Verification items for the finished model (mm, model axes). A direction names the side the tool comes from. Round coordinates to 2 decimals unless told otherwise and drop trailing zeros. Order: outer loops, then holes, each group sorted by start corner. A loop starts at its lowest first (then second) coordinate and runs counter-clockwise, first axis right, second up. Notation, with made-up numbers: (-21, 72.5) -> (34, 72.5) arc R24 ccw to (34, 85.5) -> close; hole circle Ø8 at (83.25, -13.5). An arc over 180 degrees is marked (long way). Return JSON: item names as keys, results as strings. Group by question number.
1) Section check A-A on x = 0. Enter the section's corners in (y, z).
2) Depth check by flat-ended pin: pin 1 (6 mm diameter, centred on y = -4.5, z = 8.5, fed in from -X); pin 2 (2.5 mm diameter, centred on x = -9, y = -0.5, fed in from +Z); pin 3 (0.8 mm diameter, centred on y = -9.5, z = 9.5, fed in from -X). Enter the tip coordinate at first touch or a pass-through.
3) Draft check along Y on faces 4 (the cylindrical face through (1.9, 11.59, 7.57)), 5 (the cylindrical face through (-3.47, -15.62, 4.45)), 6 (the flat face through (-11, -1, 7)). Enter one of: pulls with the +Y half, pulls with the -Y half, needs draft (parallel to the pull), parting line crosses it, or undercut.
4) Scan lines: L1, parallel to Y at x = 0, z = 3; L2, parallel to X at y = -1, z = 5.75; L3, parallel to X at y = -1, z = 8.75. Record each from-to range of solid material in increasing order.
5) Tool access check on faces 1 (the cylindrical face through (-12.5, 0.1, 8.5)), 2 (the cylindrical face through (-11, 0, 4)), 3 (the flat face through (-2.5, -11.4, 9.5)). Record the directions out of +Z, -Z, +X, -X, +Y, -Y that give a thin tool (end or side, any length) a straight path to the whole face; none if there is none.
6) Section check B-B on z = 7.5. Enter the section's corners in (x, y).
```python
from build123d import *

# Parameters (mm, degrees)
SKETCH_R        = 16
SKETCH_R_2      = 7.5
PAD_DEPTH       = 10
SKETCH001_R     = 1.5
POCKET_DEPTH    = 10.001
SKETCH002_W     = 5
SKETCH002_H     = 40
POCKET001_DEPTH = 3
FILLET_R        = 2
FILLET001_R     = 2
CHAMFER_SIZE    = 1
SKETCH003_R     = 3
POCKET002_DEPTH = 3


with BuildPart() as part:
    # Sketch → Pad (new body)
    with BuildSketch(Plane.XY):
        Circle(SKETCH_R)
        Circle(SKETCH_R_2, mode=Mode.SUBTRACT)
    extrude(amount=PAD_DEPTH)

    # Sketch001 (on Face4 of Pad) → Pocket (cut, through all)
    with BuildSketch(Plane.XY.offset(10)):
        with Locations((9.5, 0)):
            Circle(SKETCH001_R)
        with Locations((-9.5, 0)):
            Circle(SKETCH001_R)
    extrude(amount=-POCKET_DEPTH, mode=Mode.SUBTRACT)

    # Sketch002 (on Face3 of Pocket) → Pocket001 (cut)
    with BuildSketch(Plane.XY.offset(10)):
        Rectangle(SKETCH002_W, SKETCH002_H)
    extrude(amount=-POCKET001_DEPTH, mode=Mode.SUBTRACT)

    # Fillet
    fillet_edges = [part.edges().sort_by_distance(p)[0] for p in [
        (-2.5, 11.437274, 7),
        (2.5, 11.437274, 7),
        (2.5, -11.437274, 7),
        (-2.5, -11.437274, 7),
    ]]
    fillet(fillet_edges, radius=FILLET_R)

    # Fillet001
    fillet001_edges = [part.edges().sort_by_distance(p)[0] for p in [
        (12.165525, -10.392305, 10),
        (12.165525, 10.392305, 10),
        (-16, 0, 10),
    ]]
    fillet(fillet001_edges, radius=FILLET001_R)

    # Chamfer
    chamfer_edges = [part.edges().sort_by_distance(p)[0] for p in [
        (-16, 0, 0),
    ]]
    chamfer(chamfer_edges, length=CHAMFER_SIZE)

    # Sketch003 (on Face19 of Chamfer) → Pocket002 (cut)
    with BuildSketch(Plane.XY.offset(10)):
        with Locations((-9.5, 0)):
            Circle(SKETCH003_R)
        with Locations((9.5, 0)):
            Circle(SKETCH003_R)
    extrude(amount=-POCKET002_DEPTH, mode=Mode.SUBTRACT)


solid = part.part
```
Check result:
{
 "1": {"outline": "(-16, 1) -> (-15, 0) -> (-7.5, 0) -> (-7.5, 7) -> (-16, 7) -> close; (7.5, 0) -> (15, 0) -> (16, 1) -> (16, 7) -> (7.5, 7) -> close"},
 "2": {"pin 1": "x = -15.93", "pin 2": "z = 7", "pin 3": "x = -12.57"},
 "3": {"face 4": "needs draft", "face 5": "parting line crosses it", "face 6": "undercut"},
 "4": {"L1": "-16 to -7.5, 7.5 to 16", "L2": "-15.97 to -10.62, -8.38 to -7.43, 7.43 to 8.38, 10.62 to 15.97", "L3": "-15.82 to -12.33, 12.33 to 15.82"},
 "5": {"face 1": "+Z", "face 2": "+Z, -Z", "face 3": "+Z, +Y, -Y"},
 "6": {"outline": "(-7.24, -1.97) arc R3 cw (long way) to (-7.24, 1.97) arc R7.5 cw to (-1.82, 7.28) -> (-1.82, 15.9) arc R16 ccw to (-1.82, -15.9) -> (-1.82, -7.28) arc R7.5 cw to start; (1.82, -15.9) arc R16 ccw to (1.82, 15.9) -> (1.82, 7.28) arc R7.5 cw to (7.24, 1.97) arc R3 cw (long way) to (7.24, -1.97) arc R7.5 cw to (1.82, -7.28) -> close"}
}
